from build123d import *

# Parameters (mm, degrees)
PAD_DEPTH    = 10
SKETCH001_R  = 1.6
POCKET_DEPTH = 3


with BuildPart() as part:
    # Sketch → Pad (new body)
    with BuildSketch(Plane.YZ):
        Polygon((-9, -15), (0, -15), (0, -25), (12, -25), (12, -15), (21, -15), (21, -18), (14, -18), (14, -27), (-2, -27), (-2, -18), (-9, -18), align=None)
    extrude(amount=PAD_DEPTH)

    # Sketch001 (on Face1 of Pad) → Pocket (cut)
    with BuildSketch(Plane(origin=(0, 0, -15), x_dir=(0, -1, 0), z_dir=(0, 0, 1))):
        with Locations((6, 5)):
            Circle(SKETCH001_R)
        with Locations((-18, 5)):
            Circle(SKETCH001_R)
    extrude(amount=-POCKET_DEPTH, mode=Mode.SUBTRACT)


solid = part.part
CAD build for the part. Positions are in the model's coordinates, mm. A direction names the side the tool comes from. Round coordinates to 2 decimals unless told otherwise and drop trailing zeros. Order: outer loops, then holes, each group sorted by start corner. A loop starts at its lowest first (then second) coordinate and runs counter-clockwise, first axis right, second up. Notation, with made-up numbers: (25, 34) -> (60, 34) arc R25 cw to (60, 50) -> close; hole circle Ø8 at (57, 40). An arc over 180 degrees is marked (long way). Write item = value, one per line. Start each with the question number.
(1) Cut at C-C, the plane x = 2.5. List the corners of the cut face in (y, z).
(2) Pin check, flat tips, straight feed: P1, Ø4, axis at x = 5, y = -6, coming from the -Z side; P2, Ø2.5, axis at x = 5, z = -21.5, coming from the -Y side; P3, Ø1.5, axis at x = 7.5, z = -25, coming from the +Y side. Stop position of each tip, or through.
(3) Cut at A-A, the plane y = 18. List the corners of the cut face in (x, z), then the cut area to 3 significant figures.
(4) Cut at D-D, the plane z = -25.75. List the corners of the cut face in (x, y), then the cut area to 3 significant figures.
(5) Probe line 1 (Y direction, x = 3.75, z = -20.25); line 2 (X direction, y = -6, z = -16.6); line 3 (Z direction, x = 8.75, y = 10). List the from-to ranges inside material, lowest first. Write a range as [from, to].
(6) Pull direction X, two halves, no side cores. Call faces 1 (the flat face through (10, 6, -26)), 2 (the cylindrical face through (4.03, 19.27, -16.48)), 3 (the flat face through (5, -4, -15)): released by +X, released by -X, zero draft, split by the parting line, or undercut.
(7) Which spindle directions (+Z, -Z, +X, -X, +Y, -Y) get a long thin tool onto all of the face, cutting with end or side? Do faces 4 (the flat face through (5, 16, -18)), 5 (the flat face through (3.8, -4.7, -18)), 6 (the flat face through (5, 0, -20)). Say none if no direction does.
(8) Cut at B-B, the plane x = 5. List the corners of the cut face in (y, z), then the cut area to 3 significant figures.
Model answer:
q1.outline = (-9, -18) -> (-2, -18) -> (-2, -27) -> (14, -27) -> (14, -18) -> (21, -18) -> (21, -15) -> (12, -15) -> (12, -25) -> (0, -25) -> (0, -15) -> (-9, -15) -> close
q2.P1 = -18
q2.P2 = -2
q2.P3 = 14
q3.outline = (0, -18) -> (3.4, -18) -> (3.4, -15) -> (0, -15) -> close; (6.6, -18) -> (10, -18) -> (10, -15) -> (6.6, -15) -> close
q3.area = 20.4 mm2
q4.outline = (0, -2) -> (10, -2) -> (10, 14) -> (0, 14) -> close
q4.area = 160 mm2
q5.line_1 = [-2, 0], [12, 14]
q5.line_2 = [0, 3.4], [6.6, 10]
q5.line_3 = [-27, -25]
q6.face_1 = released by +X
q6.face_2 = undercut
q6.face_3 = zero draft
q7.face_4 = -Z, +X, -X, +Y
q7.face_5 = -Z, +X, -X, -Y
q7.face_6 = +Z, +X, -X
q8.outline = (-9, -18) -> (-7.6, -18) -> (-7.6, -15) -> (-9, -15) -> close; (-4.4, -18) -> (-2, -18) -> (-2, -27) -> (14, -27) -> (14, -18) -> (16.4, -18) -> (16.4, -15) -> (12, -15) -> (12, -25) -> (0, -25) -> (0, -15) -> (-4.4, -15) -> close; (19.6, -18) -> (21, -18) -> (21, -15) -> (19.6, -15) -> close
q8.area = 94.8 mm2
